```python
from build123d import *

# Parameters (mm, degrees)
BOSS_EXTRU_1_DEPTH = 5
CONG_1_R           = 10


with BuildPart() as part:
    # Esquisse1 → Boss.-Extru.1 (new body)
    with BuildSketch(Plane.XY):
        Polygon((15, 0), (27.5, 12.5), (27.5, 20), (22.5, 20), (22.5, 25), (17.5, 25), (17.5, 20), (14, 20), (14, 17), (15.1, 17), (15.1, 14.7), (14, 14.7), (14, 10), (11, 10), (11, 14.7), (9.9, 14.7), (9.9, 17), (11, 17), (11, 20), (7.5, 20), (7.5, 25), (2.5, 25), (2.5, 20), (-2.5, 20), (-2.5, 25), (-7.5, 25), (-7.5, 20), (-11, 20), (-11, 17), (-9.9, 17), (-9.9, 14.7), (-11, 14.7), (-11, 10), (-14, 10), (-14, 14.7), (-15.1, 14.7), (-15.1, 17), (-14, 17), (-14, 20), (-17.5, 20), (-17.5, 25), (-22.5, 25), (-22.5, 20), (-27.5, 20), (-27.5, 12.5), (-15, 0), (-10, 0), (-10, -5), (-5, -5), (-5, 0), (-1.5, 0), (-1.5, 3), (-2.6, 3), (-2.6, 5.3), (-1.5, 5.3), (-1.5, 10), (1.5, 10), (1.5, 5.3), (2.6, 5.3), (2.6, 3), (1.5, 3), (1.5, 0), (5, 0), (5, -5), (10, -5), (10, 0), align=None)
    extrude(amount=BOSS_EXTRU_1_DEPTH)

    # Congé1
    cong_1_edges = [part.edges().sort_by_distance(p)[0] for p in [
        (27.5, 12.5, 2.5),
        (-27.5, 12.5, 2.5),
    ]]
    fillet(cong_1_edges, radius=CONG_1_R)


solid = part.part
```
Read the model definition and answer for the solid it produces. Units are mm, in the model's axes. A direction names the side the tool comes from. Coordinates: 2 decimals unless noted, no trailing zeros. Write each loop counter-clockwise with the first axis right and the second up, starting at its lowest first coordinate (ties: lowest second). Pieces come first, ordered by that corner, then holes. Notation, with made-up numbers: (22, 45) -> (73, 45) arc R23 ccw to (73, 65) -> close; hole circle Ø9 at (-32, -27.75). An arc over 180 degrees is marked (long way). Return JSON: item names as keys, results as strings.
1. A cutting plane is placed at B-B (y = 11.5). Determine the outline of the cut face in (x, z).
Found:
{"outline": "(-26.08, 0) -> (-14, 0) -> (-14, 5) -> (-26.08, 5) -> close; (-11, 0) -> (11, 0) -> (11, 5) -> (-11, 5) -> close; (14, 0) -> (26.08, 0) -> (26.08, 5) -> (14, 5) -> close"}
2. Find the intervals of material crossed by line 1 along X through (y, z) = (17.5, 2.6); line 2 along X through (y, z) = (20.75, 1.35); line 3 along X through (y, z) = (16.5, 2.75), in increasing order. Write a range as from..to.
Found:
{"line 1": "-27.5..-14, -11..11, 14..27.5", "line 2": "-22.5..-17.5, -7.5..-2.5, 2.5..7.5, 17.5..22.5", "line 3": "-27.5..-15.1, -9.9..9.9, 15.1..27.5"}
3. A cutting plane is placed at D-D (x = -13). Determine the outline of the cut face in (y, z), and give its area (3 significant figures).
Found:
{"outline": "(0, 0) -> (10, 0) -> (10, 5) -> (0, 5) -> close", "area": "50.0 mm2"}
4. Each of these flat-tipped pins is pushed along its axis until it touches: P1, Ø1, axis at x = 8.5, z = 3, coming from the +Y side; P2, Ø2.5, axis at y = 4.5, z = 3.5, coming from the +X side; P3, Ø2, axis at y = 3.5, z = 2, coming from the +X side. Where does it stop, or does it pass through?
Found:
{"P1": "y = 20", "P2": "x = 20.75", "P3": "x = 19.5"}
5. Determine the mould class of faces 1 (the face through (14.5, 17, 2.5)), 2 (the face through (-26.76, 12.87, 2.54)), 3 (the face through (22.5, 22, 2)) for opening direction X: pulls with the +X half, pulls with the -X half, needs draft (parallel to the pull), parting line crosses it, or undercut.
Found:
{"face 1": "undercut", "face 2": "pulls with the -X half", "face 3": "pulls with the +X half"}
6. A cutting plane is placed at A-A (y = 22.5). Determine the outline of the cut face in (x, z), and give its area (3 significant figures).
Found:
{"outline": "(-22.5, 0) -> (-17.5, 0) -> (-17.5, 5) -> (-22.5, 5) -> close; (-7.5, 0) -> (-2.5, 0) -> (-2.5, 5) -> (-7.5, 5) -> close; (2.5, 0) -> (7.5, 0) -> (7.5, 5) -> (2.5, 5) -> close; (17.5, 0) -> (22.5, 0) -> (22.5, 5) -> (17.5, 5) -> close", "area": "100 mm2"}
7. A tool of negligible diameter and unlimited length cuts with its end or side. For faces 4 (the face through (10.5, 14.7, 2.5)), 5 (the face through (10, -3, 2)), 6 (the face through (-12, 10, 2)), 7 (the face through (-5, -3, 2)), 8 (the face through (25, 20, 2)), from which of +Z, -Z, +X, -X, +Y, -Y can it reach the whole face along a straight path? Write none if from no direction.
Found:
{"face 4": "+Z, -Z", "face 5": "+Z, -Z, +X, -Y", "face 6": "+Z, -Z, +Y", "face 7": "+Z, -Z, -Y", "face 8": "+Z, -Z, +X, +Y"}
8. A cutting plane is placed at C-C (x = 19.5). Determine the outline of the cut face in (y, z).
Found:
{"outline": "(4.5, 0) -> (25, 0) -> (25, 5) -> (4.5, 5) -> close"}
